Solid Edge part; units mm, degrees
sketch "Sketch1" plane through (0, 0, 0) normal (0, 0, -1) x (-1, 0, 0)
  arc A0 (3.9382, 6.3828) -> (1.7286, 7.2981) centre (0, 0) ccw
  arc A1 (1.7286, 7.2981) -> (-1.7286, 7.2981) centre (0, 9.75) cw
  arc A2 (-1.7286, 7.2981) -> (-3.9382, 6.3828) centre (0, 0) ccw
  arc A3 (-3.9382, 6.3828) -> (-6.3828, 3.9382) centre (-6.8943, 6.8943) cw
  arc A4 (-6.3828, 3.9382) -> (-7.2981, 1.7286) centre (0, 0) ccw
  arc A5 (-7.2981, 1.7286) -> (-7.2981, -1.7286) centre (-9.75, 0) cw
  arc A6 (-7.2981, -1.7286) -> (-6.3828, -3.9382) centre (0, 0) ccw
  arc A7 (-6.3828, -3.9382) -> (-3.9382, -6.3828) centre (-6.8943, -6.8943) cw
  arc A8 (-3.9382, -6.3828) -> (-1.7286, -7.2981) centre (0, 0) ccw
  arc A9 (-1.7286, -7.2981) -> (1.7286, -7.2981) centre (0, -9.75) cw
  arc A10 (1.7286, -7.2981) -> (3.9382, -6.3828) centre (0, 0) ccw
  arc A11 (3.9382, -6.3828) -> (6.3828, -3.9382) centre (6.8943, -6.8943) cw
  arc A12 (6.3828, -3.9382) -> (7.2981, -1.7286) centre (0, 0) ccw
  arc A13 (7.2981, -1.7286) -> (7.2981, 1.7286) centre (9.75, 0) cw
  arc A14 (7.2981, 1.7286) -> (6.3828, 3.9382) centre (0, 0) ccw
  arc A15 (6.3828, 3.9382) -> (3.9382, 6.3828) centre (6.8943, 6.8943) cw
  circle A16 centre (0, 0) radius 1.75
extrude "Protrusion1" add sketch "Sketch1" along normal blind 4
sketch "Sketch2" plane through (0, 0, -4) normal (0, 0, -1) x (1, 0, 0)
  line L0 (2.8, 1.6166) -> (0, 3.2332)
  line L1 (0, 3.2332) -> (-2.8, 1.6166)
  line L2 (-2.8, 1.6166) -> (-2.8, -1.6166)
  line L3 (-2.8, -1.6166) -> (0, -3.2332)
  line L4 (0, -3.2332) -> (2.8, -1.6166)
  line L5 (2.8, -1.6166) -> (2.8, 1.6166)
extrude "ExtrudedCutout_1" cut sketch "Sketch2" against normal blind 2.5
The model under review builds one solid part; all positions refer to its coordinate system, in mm. A direction names the side the tool comes from. Round coordinates to 2 decimals unless told otherwise and drop trailing zeros. Loops run counter-clockwise (first coordinate to the right, second up) from the corner with the lowest first, then second, coordinate; pieces in that order, holes last. Notation, with made-up numbers: M 0,77 L 27,77 A17 ccw 27,92 Z; hole C -8.5,-38.5 d11. An arc over 180 degrees is marked long. Answer as CSV lines item,"result".
1. For faces 1 (the face through (1.42, -2.414, -2.768)), 2 (the face through (0.03, -6.75, -1.97)), list the 3-axis set-ups (+Z, -Z, +X, -X, +Y, -Y) from which the entire face can be reached by the end or side of a thin tool; tool diameter is ignored.
Outcome:
face 1,"-Z"
face 2,"+Z, -Z, -Y"
2. We need section A-A (z = -0.25). Give the boundary of the cut face in (x, y).
Outcome:
outline,"M -7.3,-1.73 A7.5 ccw -6.38,-3.94 A3 cw -3.94,-6.38 A7.5 ccw -1.73,-7.3 A3 cw 1.73,-7.3 A7.5 ccw 3.94,-6.38 A3 cw 6.38,-3.94 A7.5 ccw 7.3,-1.73 A3 cw 7.3,1.73 A7.5 ccw 6.38,3.94 A3 cw 3.94,6.38 A7.5 ccw 1.73,7.3 A3 cw -1.73,7.3 A7.5 ccw -3.94,6.38 A3 cw -6.38,3.94 A7.5 ccw -7.3,1.73 A3 cw Z; hole C 0,0 d3.5"
3. We need section D-D (y = 2.25). Give the boundary of the cut face in (x, z), plus the area to 3 significant figures.
Outcome:
outline,"M -7.15,-4 L -1.7,-4 L -1.7,-1.5 L 1.7,-1.5 L 1.7,-4 L 7.15,-4 L 7.15,0 L -7.15,0 Z"
area,"48.7 mm2"
4. We need section B-B (y = 0). Give the boundary of the cut face in (x, z), plus the area to 4 significant figures.
Outcome:
outline,"M -6.75,-4 L -2.8,-4 L -2.8,-1.5 L -1.75,-1.5 L -1.75,0 L -6.75,0 Z; M 1.75,-1.5 L 2.8,-1.5 L 2.8,-4 L 6.75,-4 L 6.75,0 L 1.75,0 Z"
area,"34.75 mm2"
5. Insertion check: pin 1 Ø3 at (x, y) = (0, 0) entering from -Z; pin 2 Ø0.8 at (y, z) = (-0.5, -3) entering from -X. Each pin has a flat end and moves straight along its axis. Give the tip position at first contact, or say it passes through.
Outcome:
pin 1,"passes through"
pin 2,"stops at x = -6.89"
6. Draft analysis for pull direction Y (two halves, no side actions). For faces 3 (the face through (-4.791, 4.755, -1.972)), 4 (the face through (-6.75, -0.03, -1.97)), 5 (the face through (-2.89, -6.92, -1.97)), state which applies: pulls with the +Y half, pulls with the -Y half, needs draft (parallel to the pull), parting line crosses it, or undercut.
Outcome:
face 3,"pulls with the +Y half"
face 4,"undercut"
face 5,"pulls with the -Y half"
7. To check wall thickness, follow L1, parallel to Y at x = 0, z = -1.1; L2, parallel to X at y = 2.25, z = -1.7. State the ranges of each line that lie inside material, in increasing order. Write a range as [from, to].
Outcome:
L1,"y = [-6.75, -1.75], [1.75, 6.75]"
L2,"x = [-7.15, -1.7], [1.7, 7.15]"
8. We need section C-C (x = 0.5). Give the boundary of the cut face in (y, z).
Outcome:
outline,"M -6.79,-4 L -2.94,-4 L -2.94,-1.5 L -1.68,-1.5 L -1.68,0 L -6.79,0 Z; M 1.68,-1.5 L 2.94,-1.5 L 2.94,-4 L 6.79,-4 L 6.79,0 L 1.68,0 Z"
